Geometry check sheet. Reference: the model listing, model coordinates, mm. A direction names the side the tool comes from. Round coordinates to 2 decimals unless told otherwise and drop trailing zeros. Write each loop counter-clockwise with the first axis right and the second up, starting at its lowest first coordinate (ties: lowest second). Pieces come first, ordered by that corner, then holes.
Item 1: Scan lines: probe 1 along Y at (x, z) = (-40.75, 112); probe 2 along X at (y, z) = (10, 170); probe 3 along Z at (x, y) = (-39.75, 14.5). Record each from-to range of solid material in increasing order.
Item 2: Draft check along X on faces 3 (the face through (-38.216, 11, 127)), 4 (the face through (-41, 7.902, 123)), 5 (the face through (-44.716, 11, 123)). Enter one of: pulls with the +X half, pulls with the -X half, needs draft (parallel to the pull), parting line crosses it, or undercut.
Item 3: Depth check by flat-ended pin: P1, Ø0.5, axis at x = -38, z = 126.5, coming from the +Y side. Enter the tip coordinate at first touch or a pass-through.
Item 4: Access from +Z, -Z, +X, -X, +Y, -Y to the whole of each face (thin tool, end or side, straight path). Record for faces 1 (the face through (-41, 15.402, 189)), 2 (the face through (-41, 14.402, 61)).
Item 5: Cross-section at A-A (z = 87). Enter the section's corners in (x, y), then the cut area to 3 significant figures.
Item 6: Cross-section at B-B (z = 126). Enter the section's corners in (x, y).
from build123d import *

# Parameters (mm, degrees)
BOSS_EXTRU_3_DEPTH      = 250
BOSS_EXTRU_3_DEPTH_BACK = 0.0001
ESQUISSE3_W             = 7.5
ESQUISSE3_H             = 7.5
ESQUISSE4_W             = 5.5
ESQUISSE4_H             = 5.5
ENL_V_MAT_EXTRU_3_DEPTH = 255.43419698
ESQUISSE6_W             = 7.5
ESQUISSE6_H             = 7.5
ENL_V_MAT_EXTRU_4_DEPTH = 3.75
TROU_TARAUD_2_561_D     = 1.778
TROU_TARAUD_2_562_D     = 1.778
PER_AGE1_START          = 14.402314812
PER_AGE1_OUTLINE_R      = 1.5
PER_AGE1_DEPTH          = 1
PER_AGE2_START          = 7.902314812
PER_AGE2_OUTLINE_R      = 1.5
PER_AGE2_DEPTH          = 1


# Read off the part's stored shape, not the designer's step: Perçage1, Perçage2
with BuildPart() as part:
    # Esquisse3 → Boss.-Extru.3 (new, two sides: drawn at the far end of the back side and taken through both)
    with BuildSketch(Plane.XY.offset(-BOSS_EXTRU_3_DEPTH_BACK)):
        with Locations((-40.965537472, 11.652314812)):
            Rectangle(ESQUISSE3_W, ESQUISSE3_H)
    extrude(amount=BOSS_EXTRU_3_DEPTH + BOSS_EXTRU_3_DEPTH_BACK)

    # Esquisse4 → Enlèv. mat.-Extru.3 (cut, through all)
    with BuildSketch(Plane.XY.offset(250)):
        with Locations((-40.965537472, 11.652314812)):
            Rectangle(ESQUISSE4_W, ESQUISSE4_H)
    extrude(amount=-ENL_V_MAT_EXTRU_3_DEPTH, mode=Mode.SUBTRACT)

    # Esquisse6 → Enlèv. mat.-Extru.4 (cut)
    with BuildSketch(Plane(origin=(0, 15.402314812, 0), x_dir=(-1, 0, 0), z_dir=(0, 1, 0))):
        with Locations((40.965537472, 124.9999)):
            Rectangle(ESQUISSE6_W, ESQUISSE6_H)
    extrude(amount=-ENL_V_MAT_EXTRU_4_DEPTH, mode=Mode.SUBTRACT)

    # Trou taraudé #2-561 (through all)
    with Locations(Plane.XZ.offset(-7.902314812)):
        with Locations((-40.965537472, 243.6), (-40.965537472, 210.9)):
            Hole(TROU_TARAUD_2_561_D / 2)

    # Trou taraudé #2-562 (through all)
    with Locations(Plane.XZ.offset(-7.902314812)):
        with Locations((-40.965537472, 38.972883346), (-40.965537472, 6.272883346)):
            Hole(TROU_TARAUD_2_562_D / 2)

    # Perçage1 outline → Perçage1 (cut)
    with BuildSketch(Plane(origin=(0, 0, 0), x_dir=(1, 0, 0), z_dir=(0, 1, 0)).offset(PER_AGE1_START)):
        with Locations((-40.965537472, -154.69838481)):
            Circle(PER_AGE1_OUTLINE_R)
        with Locations((-40.965537472, -95.30141519)):
            Circle(PER_AGE1_OUTLINE_R)
    extrude(amount=PER_AGE1_DEPTH, mode=Mode.SUBTRACT)

    # Perçage2 outline → Perçage2 (cut)
    with BuildSketch(Plane(origin=(0, 0, 0), x_dir=(1, 0, 0), z_dir=(0, 1, 0)).offset(PER_AGE2_START)):
        with Locations((-40.965537472, -154.69838481)):
            Circle(PER_AGE2_OUTLINE_R)
        with Locations((-40.965537472, -95.30141519)):
            Circle(PER_AGE2_OUTLINE_R)
    extrude(amount=PER_AGE2_DEPTH, mode=Mode.SUBTRACT)


solid = part.part
Resolved:
1. probe 1: y = 7.9 to 8.9, 14.4 to 15.4
1. probe 2: x = -44.72 to -43.72, -38.22 to -37.22
1. probe 3: z = 0 to 94.42, 96.18 to 121.25, 128.75 to 153.82, 155.58 to 250
2. face 3: undercut
2. face 4: needs draft
2. face 5: pulls with the -X half
3. P1: stops at y = 11.65
4. face 1: +Z, -Z, +X, -X, +Y
4. face 2: +Z, -Z
5. outline: (-44.72, 7.9) - (-37.22, 7.9) - (-37.22, 15.4) - (-44.72, 15.4) - close; hole (-43.72, 8.9) - (-38.22, 8.9) - (-38.22, 14.4) - (-43.72, 14.4) - close
5. area: 26.0 mm2
6. outline: (-44.72, 7.9) - (-37.22, 7.9) - (-37.22, 11.65) - (-38.22, 11.65) - (-38.22, 8.9) - (-43.72, 8.9) - (-43.72, 11.65) - (-44.72, 11.65) - close
